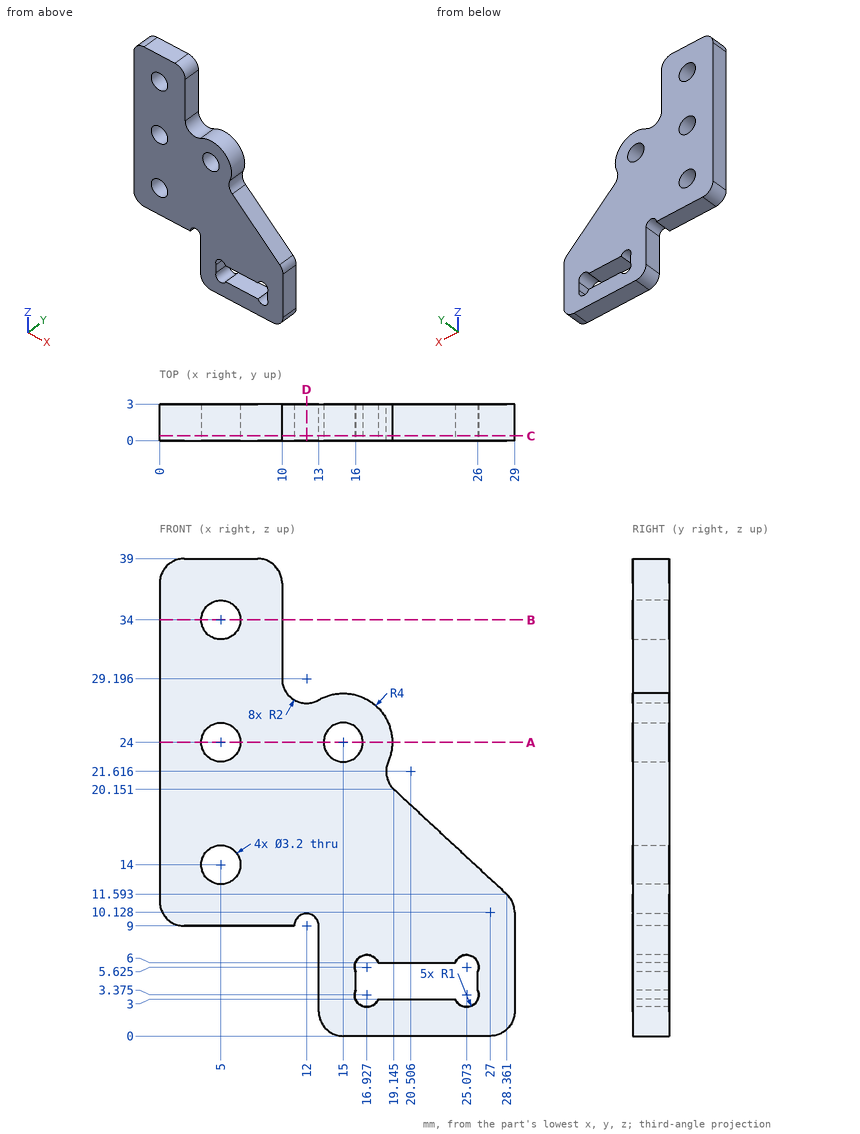
Part print with two shaded views. Sizes in mm from the minimum x, y, z corner. Give positions to 0.01 mm unless a question says otherwise; leave off trailing zeros. Loops run counter-clockwise (first coordinate to the right, second up) from the corner with the lowest first, then second, coordinate; pieces in that order, holes last. Notation, with made-up numbers: (-7, 39.5) - (46, 39.5) arc R21 ccw to (46, 44.5) - close; hole circle Ø7 at (69.5, 82.5). An arc over 180 degrees is marked (long way). Put each result on its own line as item: value.
Q1. Slice it at A-A (z = 24). Give the cut face in (x, y).
Filled in:
outline: (0, 0) - (3.4, 0) - (3.4, 3) - (0, 3) - close; (6.6, 0) - (13.4, 0) - (13.4, 3) - (6.6, 3) - close; (16.6, 0) - (19, 0) - (19, 3) - (16.6, 3) - close
Q2. Slice it at B-B (z = 34). Give the cut face in (x, y).
Filled in:
outline: (0, 0) - (3.4, 0) - (3.4, 3) - (0, 3) - close; (6.6, 0) - (10, 0) - (10, 3) - (6.6, 3) - close
Q3. Slice it at C-C (y = 0.4). Give the number of separate pieces and of enclosed holes in the cut face.
Filled in:
separate pieces: 1
enclosed holes: 5
Q4. Slice it at D-D (x = 12). Give the cut face in (y, z).
Filled in:
outline: (0, 10) - (3, 10) - (3, 27.2) - (0, 27.2) - close
Q5. Probe line 1 along X through (y, z) = (1.55, 24); line 2 along Z through (x, y) = (5.75, 2) (1 decimal); line 3 along X through (y, z) = (0.9, 34). List the from-to ranges inside material, lowest first.
Filled in:
line 1: x = 0 to 3.4, 6.6 to 13.4, 16.6 to 19
line 2: z = 9 to 12.6, 15.4 to 22.6, 25.4 to 32.6, 35.4 to 39
line 3: x = 0 to 3.4, 6.6 to 10
Q6. Flat gauge pins, fed straight in: pin 1 (1.5 mm diameter, centred on x = 6, y = 1, fed in from -Z); pin 2 (1.2 mm diameter, centred on y = 2, z = 4.5, fed in from -X); pin 3 (1.9 mm diameter, centred on x = 5, z = 14, fed in from -Y); pin 4 (0.9 mm diameter, centred on x = 19.5, y = 1, fed in from +Z) (1 decimal). Where does each tip first touch, or does it go through?
Filled in:
pin 1: stops at z = 9
pin 2: stops at x = 13
pin 3: passes through
pin 4: stops at z = 20.2
